Build history of the part. All positions in model axes, mm. A direction names the side the tool comes from. Give positions to 0.01 mm unless a question says otherwise; leave off trailing zeros. Order: outer loops, then holes, each group sorted by start corner. A loop starts at its lowest first (then second) coordinate and runs counter-clockwise, first axis right, second up. Notation, with made-up numbers: (-24, 8) - (12, 8) arc R17 cw to (12, 20) - close; hole circle Ø10 at (31, 35). An arc over 180 degrees is marked (long way). Use a Markdown table: item, result.
Autodesk Inventor part; units mm, degrees
ref_plane "YZ Plane" through (0, 0, 0) normal (1, 0, 0) x (0, 1, 0)
ref_plane "XZ Plane" through (0, 0, 0) normal (0, 1, 0) x (-1, 0, 0)
ref_plane "XY Plane" through (0, 0, 0) normal (0, 0, 1) x (1, 0, 0)
sketch "Skizze1" plane through (0, 0, 0) normal (0, 0, 1) x (1, 0, 0)
  line L0 (-16, 16) -> (16, 16)
  line L1 (16, 16) -> (16, -16)
  line L2 (16, -16) -> (-16, -16)
  line L3 (-16, -16) -> (-16, 16)
  line L4 (0, 22.4) -> (0, -22.4)
  line L5 (-22.4, 0) -> (22.4, 0)
  point P0 (0, 0)
  dimension "d0" = 32
  dimension "d1" = 32
extrude "Extrusion1" add sketch "Skizze1" along normal mid plane 6
sketch "Skizze2" plane through (0, 0, 0) normal (0, 0, 1) x (1, 0, 0)
  line L0 (-16, 16) -> (-16, -16)
  line L1 (-16, -16) -> (-26.5, -16)
  line L2 (-26.5, -16) -> (-26.5, -13)
  line L3 (-26.5, -13) -> (-16, -13)
  line L4 (-16, -13) -> (-16, -16)
  line L5 (0, 22.4) -> (0, -22.4)
  line L6 (16, -16) -> (26.5, -16)
  line L7 (26.5, -16) -> (26.5, -13)
  line L8 (26.5, -13) -> (16, -13)
  line L9 (16, -13) -> (16, -16)
  point P0 (0, 0)
  dimension "d6" = 10.5
  dimension "d7" = 3
extrude "Extrusion2" add sketch "Skizze2" along normal mid plane 6
fillet "Rundung1" radius 16 2 edges at (-16, 16, 0) (16, 16, 0)
fillet "Rundung2" radius 1 2 edges at (-16, -13, 0) (16, -13, 0)
sketch "Skizze3" plane through (0, 0, 3) normal (0, 0, 1) x (1, 0, 0)
  circle A0 centre (0, 0) radius 7.6
  dimension "d12" = 15.2
extrude "Extrusion3" cut sketch "Skizze3" against normal blind 4
sketch "Skizze4" plane through (0, 0, -1) normal (0, 0, 1) x (1, 0, 0)
  circle A0 centre (0, 0) radius 6
  dimension "d15" = 12
extrude "Extrusion4" cut sketch "Skizze4" against normal up to surface (2 mm away)
sketch "Skizze5" plane through (-26.5, -13, 3) normal (0, 1, 0) x (1, 0, 0)
  circle A0 centre (3.5, 3) radius 1.6
  circle A1 centre (49.5, 3) radius 1.6
  line L0 (0, 6) -> (9.5, 6)
  line L1 (0, 6) -> (0, 0)
  line L2 (53, 6) -> (53, 0)
  line L3 (43.5, 6) -> (53, 6)
  point P0 (26.5, 3)
  dimension "d18" = 3.2
  dimension "d19" = 3.2
  dimension "d20" = 3
  dimension "d21" = 3.5
  dimension "d22" = 3.5
  dimension "d23" = 3
extrude "Extrusion5" cut sketch "Skizze5" against normal up to surface (3 mm away)
sketch "Skizze6" plane through (-26.5, -16, 3) normal (0, -1, 0) x (1, 0, 0)
  line L0 (9.5, 0) -> (0, 0)
  line L1 (53, 0) -> (53, -6)
  line L2 (0, 0) -> (53, 0)
  line L3 (53, 0) -> (53, -6)
  line L4 (53, -6) -> (0, -6)
  line L5 (0, -6) -> (0, 0)
  circle A0 centre (3.5, -3) radius 1.6
  circle A1 centre (3.5, -3) radius 1.6
  circle A2 centre (49.5, -3) radius 1.6
  circle A3 centre (49.5, -3) radius 1.6
  point P0 (26.5, -3)
  point P1 (9.5, 0)
  dimension "d26" = 3.2
  dimension "d27" = 3.2
extrude "Extrusion6" add sketch "Skizze6" along normal blind 1.5
properties part number "_3D-Druck"
1) Slice it at A-A (z = 0). State how many separate pieces and enclosed holes the cut face has, and give its area (3 significant figures).
Computed:
| item | result |
|---|---|
| separate pieces | 3 |
| enclosed holes | 1 |
| area | 847 mm² |
2) Wall check: line 1 (Y direction, x = 0, z = -2.3); line 2 (Y direction, x = 2.5, z = -0.5); line 3 (X direction, y = -4.5, z = 1.65). Give the ranges that are in metal, low to high. Write a range as from..to.
Computed:
| item | result |
|---|---|
| line 1 | y = -17.5..-6, 6..16 |
| line 2 | y = -17.5..-7.18, 7.18..15.8 |
| line 3 | x = -16..-6.12, 6.12..16 |
3) Tool access for faces 1 (the flat face through (6, 2, -1)), 2 (the flat face through (21, -13, 0)), 3 (the flat face through (-16, -6, 0)): list every direction of +Z, -Z, +X, -X, +Y, -Y with a clear straight run to the whole face (end or side of a thin tool).
Computed:
| item | result |
|---|---|
| face 1 | +Z |
| face 2 | +Z, -Z, +X, +Y |
| face 3 | +Z, -Z, -X, +Y |
4) Pin check, flat tips, straight feed: P1, Ø3, axis at y = -6, z = -1, coming from the +X side; P2, Ø1, axis at x = 6.5, z = -2, coming from the +Y side. Stop position of each tip, or through.
Computed:
| item | result |
|---|---|
| P1 | stops at x = 16 |
| P2 | stops at y = 14.83 |
5) Slice it at D-D (y = 9.5). Write the cut outline in (x, z).
Computed:
| item | result |
|---|---|
| outline | (-12.87, -3) - (12.87, -3) - (12.87, 3) - (-12.87, 3) - close |
6) Slice it at B-B (x = 23). Write the cut outline in (y, z).
Computed:
| item | result |
|---|---|
| outline | (-17.5, -3) - (-13, -3) - (-13, -1.6) - (-17.5, -1.6) - close; (-17.5, 1.6) - (-13, 1.6) - (-13, 3) - (-17.5, 3) - close |
7) Two-plate mould, pull along Y, no slides. Class faces 4 (the flat face through (0, -17.5, 0)), 5 (the cylindrical face through (-16.301, -12.715, 0.042)), 6 (the cylindrical face through (-6, 0, -2)), 7 (the cylindrical face through (24.526, -15.218, -0.481)): +Y half, -Y half, draft (parallel to the pull), parting line (faces both ways), or undercut.
Computed:
| item | result |
|---|---|
| face 4 | -Y half |
| face 5 | +Y half |
| face 6 | undercut |
| face 7 | draft |
8) Slice it at C-C (x = -7). Write the cut outline in (y, z).
Computed:
| item | result |
|---|---|
| outline | (-17.5, -3) - (14.39, -3) - (14.39, 3) - (2.96, 3) - (2.96, -1) - (-2.96, -1) - (-2.96, 3) - (-17.5, 3) - close |
